from build123d import *

# Parameters (mm, degrees)
BOSS_EXTRUDE2_DEPTH = 20
CUT_EXTRUDE1_DEPTH  = 6


with BuildPart() as part:
    # Sketch1 → Boss-Extrude2 (new body)
    with BuildSketch(Plane(origin=(0, 0, 0), x_dir=(0, 0, -1), z_dir=(1, 0, 0))):
        with BuildLine():
            Line((0, 0), (-28, 0))
            Line((-28, 0), (-28, 34.803847577))
            Line((-28, 34.803847577), (-27, 34.803847577))
            ThreePointArc((-27, 34.803847577), (-14, 26), (-1, 34.803847577))
            Line((-1, 34.803847577), (0, 34.803847577))
            Line((0, 34.803847577), (0, 0))
        make_face()
    extrude(amount=-BOSS_EXTRUDE2_DEPTH)

    # Sketch3 → Cut-Extrude1 (cut)
    with BuildSketch(Plane(origin=(0, 0, 0), x_dir=(0, 0, -1), z_dir=(1, 0, 0))):
        with BuildLine():
            Line((-28, 20), (-28, 26))
            ThreePointArc((-28, 26), (-14, 17.745966692), (0, 26))
            Line((0, 26), (0, 20))
            ThreePointArc((0, 20), (-14, 14.125783199), (-28, 20))
        make_face()
    extrude(amount=-CUT_EXTRUDE1_DEPTH, mode=Mode.SUBTRACT)


solid = part.part
Verification items for the finished model (mm, model axes). A direction names the side the tool comes from. Coordinates: 2 decimals unless noted, no trailing zeros. Order: outer loops, then holes, each group sorted by start corner. A loop starts at its lowest first (then second) coordinate and runs counter-clockwise, first axis right, second up. Notation, with made-up numbers: M 55,86 L 109,86 A29 cw 109,122 Z; hole C 10.25,48 d11. An arc over 180 degrees is marked long. One line per item, written item: value. Start each with the question number.
Item 1: Sectioned sample at B-B (x = -11). Enter the section's corners in (y, z).
Item 2: Sectioned sample at C-C (y = 33). Enter the section's corners in (x, z), then the cut area to 3 significant figures.
Item 3: Access from +Z, -Z, +X, -X, +Y, -Y to the whole of each face (thin tool, end or side, straight path). Record for faces 4 (the flat face through (0, 8, 14)), 5 (the cylindrical face through (-2.958, 17.748, 14.239)).
Item 4: Sectioned sample at A-A (x = -4.5). Enter the section's corners in (y, z).
Item 5: Mould release check, pull along Z, two halves, no side actions. Record for faces 1 (the flat face through (-10, 17, 28)), 2 (the flat face through (-6, 17, 13)), 3 (the flat face through (0, 24, 14)): released by +Z, released by -Z, zero draft, split by the parting line, or undercut.
Item 6: Scan lines: probe 1 along Y at (x, z) = (-15.75, 13.75); probe 2 along Y at (x, z) = (-2.25, 20.75); probe 3 along Z at (x, y) = (-10.5, 28.5). Record each from-to range of solid material in increasing order.
Item 7: Sectioned sample at D-D (z = 19.5). Enter the section's corners in (x, y), then the cut area to 3 significant figures.
Item 8: Gauge pin test, flat end, axial feed: pin 1 (2 mm diameter, centred on x = -11.5, z = 15, fed in from +Y). Record the tip position at first contact, or that the pin passes through.
Conclusion:
1. outline: M 0,0 L 34.8,0 L 34.8,1 A14 cw 34.8,27 L 34.8,28 L 0,28 Z
2. outline: M -20,0 L 0,0 L 0,1.88 L -20,1.88 Z; M -20,26.12 L 0,26.12 L 0,28 L -20,28 Z
2. area: 75.0 mm^2
3. face 4: +Z, -Z, +X, +Y, -Y
3. face 5: +X
4. outline: M 0,0 L 20,0 A19.62 cw 20,28 L 0,28 Z; M 26,0 L 34.8,0 L 34.8,1 A14 cw 34.8,27 L 34.8,28 L 26,28 A16 ccw Z
5. face 1: released by +Z
5. face 2: undercut
5. face 3: zero draft
6. probe 1: y = 0 to 26
6. probe 2: y = 0 to 15.32, 19.24 to 27.73
6. probe 3: z = 0 to 6.02, 21.98 to 28
7. outline: M -20,0 L 0,0 L 0,14.91 L -6,14.91 L -6,18.72 L 0,18.72 L 0,27.13 L -20,27.13 Z
7. area: 520 mm^2
8. pin 1: stops at y = 26.14
